Verification items for the finished model (mm, model axes). Round coordinates to 2 decimals unless told otherwise and drop trailing zeros. Order: outer loops, then holes, each group sorted by start corner. A loop starts at its lowest first (then second) coordinate and runs counter-clockwise, first axis right, second up.
```python
from build123d import *

# Parameters (mm, degrees)
F1_DEPTH       = 3
F3_D           = 3.3
F3_DEPTH       = 14.4
F3_CBORE_D     = 6.5
F3_CBORE_DEPTH = 3
F3_TIP         = 0.9914200214


with BuildPart() as f1:
    # F0 (on Front) → F1 (new body)
    with BuildSketch(Plane.XZ):
        with BuildLine():
            Line((52.4541210128, 6.1781848239), (-22.3743356764, 6.1781848239))
            Line((-22.3743356764, 6.1781848239), (-22.3743356764, -14.0438194092))
            Line((-22.3743356764, -14.0438194092), (52.5663935712, -14.0438194092))
            ThreePointArc((52.5663935712, -14.0438194092), (61.0848860922, -9.2816896986), (61.4901453485, 0.469123557))
            Line((61.4901453485, 0.469123557), (61.3778727901, 0.6911277901))
            ThreePointArc((61.3778727901, 0.6911277901), (57.6919913022, 4.696677345), (52.4541210128, 6.1781848239))
        make_face()
    extrude(amount=F1_DEPTH)

    # F3
    with Locations(Plane(origin=(0, 0, 0), x_dir=(-1, 0, 0), z_dir=(0, 1, 0))):
        with Locations((-31.9307483733, -4.7722645104), (-4.6180379577, -4.7722645104)):
            CounterBoreHole(F3_D / 2, F3_CBORE_D / 2, F3_CBORE_DEPTH, depth=F3_DEPTH)
            with Locations((0, 0, -(F3_DEPTH + F3_TIP / 2))):  # 118° drill point
                Cone(0, F3_D / 2, F3_TIP, mode=Mode.SUBTRACT)


solid = f1.part
```
1) Sectioned sample at B-B on y = -1.3. Record the cut outline in (x, z).
2) Sectioned sample at A-A on z = -6.5. Record the cut outline in (x, y), then the cut area to 3 significant figures.
3) Go/stop test with flat-tipped pins: pin 1 Ø3 at (x, z) = (26.5, 2.5) entering from +Y; pin 2 Ø4 at (x, z) = (31.93, -4.77) entering from -Y. Record where each tip stops, or that it passes through.
4) Sectioned sample at C-C on z = -11.75. Record the cut outline in (x, y).
5) Scan lines: probe 1 along X at (y, z) = (-2.2, -5.5); probe 2 along X at (y, z) = (-1.8, -2.5); probe 3 along Z at (x, y) = (31, -1.55). Record each from-to range of solid material in increasing order.
6) Draft check along X on faces 1 (the cylindrical face through (28.93, -1.48, -6.02)), 2 (the cylindrical face through (57.758, -1.479, 4.656)), 3 (the flat face through (20, -3, -4)). Enter one of: released by +X, released by -X, zero draft, split by the parting line, or undercut.
Returned:
1. outline: (-22.37, -14.04) - (52.57, -14.04) arc R10 ccw to (61.49, 0.47) - (61.38, 0.69) arc R10 ccw to (52.45, 6.18) - (-22.37, 6.18) - close; hole circle Ø6.5 at (4.62, -4.77); hole circle Ø6.5 at (31.93, -4.77)
2. outline: (-22.37, -3) - (1.87, -3) - (1.87, 0) - (-22.37, 0) - close; (7.37, -3) - (29.18, -3) - (29.18, 0) - (7.37, 0) - close; (34.68, -3) - (62.26, -3) - (62.26, 0) - (34.68, 0) - close
2. area: 221 mm2
3. pin 1: stops at y = 0
3. pin 2: passes through
4. outline: (-22.37, -3) - (58.94, -3) - (58.94, 0) - (-22.37, 0) - close
5. probe 1: x = -22.37 to 1.45, 7.79 to 28.76, 35.1 to 62.46
5. probe 2: x = -22.37 to 2.29, 6.94 to 29.61, 34.25 to 62.45
5. probe 3: z = -14.04 to -7.89, -1.66 to 6.18
6. face 1: undercut
6. face 2: released by +X
6. face 3: zero draft
